```python
from build123d import *

# Parameters (mm, degrees)
SKETCH1_R               = 29
BOSS_EXTRUDE1_DEPTH     = 75
SKETCH3_R               = 3.5
BOSS_EXTRUDE3_DEPTH     = 50
SKETCH3_4_R             = 3.5
CUT_EXTRUDE1_DEPTH      = 50
CUT_EXTRUDE2_DEPTH      = 30
CUT_EXTRUDE2_DEPTH_BACK = 30
CUT_EXTRUDE4_DEPTH      = 85.969655115


with BuildPart() as part:
    # Sketch1 → Boss-Extrude1 (new body)
    with BuildSketch(Plane(origin=(0, 0, 0), x_dir=(1, 0, 0), z_dir=(0, 1, 0))):
        Circle(SKETCH1_R)
    extrude(amount=BOSS_EXTRUDE1_DEPTH)

    # Sketch3 → Boss-Extrude3 (add)
    with BuildSketch(Plane(origin=(0, 75, 0), x_dir=(1, 0, 0), z_dir=(0, 1, 0))):
        with Locations((-21, 0)):
            Circle(SKETCH3_R)
    extrude(amount=-BOSS_EXTRUDE3_DEPTH)

    # Sketch3<4> → Cut-Extrude1 (cut)
    with BuildSketch(Plane(origin=(0, 75, 0), x_dir=(1, 0, 0), z_dir=(0, 1, 0))):
        with Locations((-21, 0)):
            Circle(SKETCH3_4_R)
    extrude(amount=-CUT_EXTRUDE1_DEPTH, mode=Mode.SUBTRACT)

    # Sketch9 → Cut-Extrude2 (cut, two sides)
    with BuildSketch(Plane.XY) as cut_extrude2_sk:
        Polygon((-12, 75), (29, 75), (29, 51.328638963), align=None)
    extrude(amount=CUT_EXTRUDE2_DEPTH, mode=Mode.SUBTRACT)
    extrude(cut_extrude2_sk.sketch, amount=-CUT_EXTRUDE2_DEPTH_BACK, mode=Mode.SUBTRACT)

    # Sketch18 → Cut-Extrude4 (cut, through all, along a direction that is not the sketch's normal)
    with BuildSketch(Plane(origin=(29.475952642, 51.053847577, 0), x_dir=(0.866025404, -0.5, 0), z_dir=(0.5, 0.866025404, 0))):
        with BuildLine():
            Line((-2.603431094, 10), (-22.603431094, 10))
            Line((-22.603431094, 10), (-22.603431094, -10))
            Line((-22.603431094, -10), (-2.603431094, -10))
            add(Edge.make_bspline(
                [(-2.603431094, -10), (1.638467326, 0), (-2.603431094, 10)],
                knots=[5.931130208, 5.931130208, 5.931130208, 6.635240406, 6.635240406, 6.635240406], degree=2, weights=[1, 0.938666041, 1]))
        make_face()
    extrude(amount=-CUT_EXTRUDE4_DEPTH, dir=(0, 1, 0), mode=Mode.SUBTRACT)


solid = part.part
```
Geometry check sheet. Reference: the model listing, model coordinates, mm. A direction names the side the tool comes from. Give positions to 0.01 mm unless a question says otherwise; leave off trailing zeros. Loops run counter-clockwise (first coordinate to the right, second up) from the corner with the lowest first, then second, coordinate; pieces in that order, holes last. Notation, with made-up numbers: (76.25, -28) - (119.25, -28) arc R16 ccw to (119.25, -4) - close; hole circle Ø4 at (52.5, 59). An arc over 180 degrees is marked (long way). Use CSV: the item, a comma, the result in double quotes. Start each with the question number.
Q1. Scan lines: probe 1 along X at (y, z) = (60, 0); probe 2 along Z at (x, y) = (0.5, 59); probe 3 along X at (y, z) = (58, -2.5). Record each from-to range of solid material in increasing order. Write a range as from..to.
Q2. Section check B-B, the plane x = 15.5. Record the cut outline in (y, z).
Q3. Access from +Z, -Z, +X, -X, +Y, -Y to the whole of each face (thin tool, end or side, straight path). Record for faces 5 (the face through (3.527, 66.035, -0.406)), 6 (the face through (9.901, 32, 0)).
Q4. Go/stop test with flat-tipped pins: pin 1 Ø1 at (y, z) = (10.5, 18.5) entering from -X; pin 2 Ø1.5 at (x, z) = (4.5, -19.5) entering from +Y; pin 3 Ø5 at (x, z) = (-20.5, 11) entering from -Y; pin 4 Ø14 at (x, y) = (18, 28) entering from +Z. Record where each tip stops, or that it passes through.
Q5. Section check D-D, the plane x = -21. Record the cut outline in (y, z).
Q6. Release check for a two-part mould opening along X. For faces 1 (the face through (16, 28, 10)), 2 (the face through (-17.66, 50.35, -1.05)), 3 (the face through (-21, 25, 0)), 4 (the face through (-28.978, 36.975, -1.132)) record: +X half, -X half, draft (parallel to the pull), parting line (faces both ways), or undercut.
Q7. Section check C-C, the plane y = 26. Record the cut outline in (x, z), and give its area (3 significant figures).
Q8. Section check A-A, the plane z = 0. Record the cut outline in (x, y).
Findings below:
1,probe 1,"x = -29..-24.5, -17.5..9.9"
1,probe 2,"z = -29..29"
1,probe 3,"x = -28.89..-23.45, -18.55..9.9"
2,outline,"(0, -24.51) - (59.12, -24.51) - (59.12, -10) - (0, -10) - close; (0, 10) - (59.12, 10) - (59.12, 24.51) - (0, 24.51) - close"
3,face 5,"+Z, -Z, +X, +Y"
3,face 6,"+X, +Y, -Y"
4,pin 1,"stops at x = -22.74"
4,pin 2,"stops at y = 65.91"
4,pin 3,"stops at y = 0"
4,pin 4,"stops at z = 26.83"
5,outline,"(0, -20) - (75, -20) - (75, -3.5) - (25, -3.5) - (25, 3.5) - (75, 3.5) - (75, 20) - (0, 20) - close"
6,face 1,"draft"
6,face 2,"undercut"
6,face 3,"undercut"
6,face 4,"parting line"
7,outline,"(9.9, -10) - (9.9, 10) - (27.22, 10) arc R29 ccw (long way) to (27.22, -10) - close; hole circle Ø7 at (-21, 0)"
7,area,"2,230 mm^2"
8,outline,"(-29, 0) - (9.9, 0) - (9.9, 62.36) - (-12, 75) - (-17.5, 75) - (-17.5, 25) - (-24.5, 25) - (-24.5, 75) - (-29, 75) - close"
